The drawing under review shows one solid part. Ordinate dimensions are in mm from its lowest x, y, z. A direction names the side the tool comes from. Coordinates: 2 decimals unless noted, no trailing zeros. Write each loop counter-clockwise with the first axis right and the second up, starting at its lowest first coordinate (ties: lowest second). Pieces come first, ordered by that corner, then holes.
Q1. To check wall thickness, follow probe 1 along X at (y, z) = (65, 14); probe 2 along X at (y, z) = (1.95, 8); probe 3 along Y at (x, z) = (93.5, 11). State the ranges of each line that lie inside material, in increasing order.
Q2. Machinability: for the marked faces 1 and 2, which of the approach directions +Z, -Z, +X, -X, +Y, -Y give a long, thin tool a straight path to every point of the face, cutting with its end or side? Answer none if there is none.
Q3. Add section A-A, the plane y = 20. Give the boundary of the cut face in (x, z), plus the area to 3 significant figures.
Q4. Add section B-B, the plane x = 40.5. Give the boundary of the cut face in (y, z), plus the area to 4 significant figures.
Q5. The part is to be moulded in two halves that separate along X. For the marked faces 3, 4 and 5, say which applies: +X half, -X half, draft (parallel to the pull), parting line (faces both ways), or undercut.
Q6. Add section C-C, the plane z = 8. Give the boundary of the cut face in (x, y).
Q7. Add section D-D, the plane z = 14.25. Give the boundary of the cut face in (x, y).
Q8. Clearance check with flat-ended pins moving along their axes: pin 1 Ø2 at (x, y) = (40.5, 63) entering from -Z; pin 2 Ø10 at (x, y) = (48.5, 30.5) entering from +Z; pin 3 Ø0.9 at (x, y) = (51, 82) entering from +Z; pin 4 Ø9 at (x, z) = (103.5, 8) entering from -Y. State where each tip first meets the part, or that it passes through.
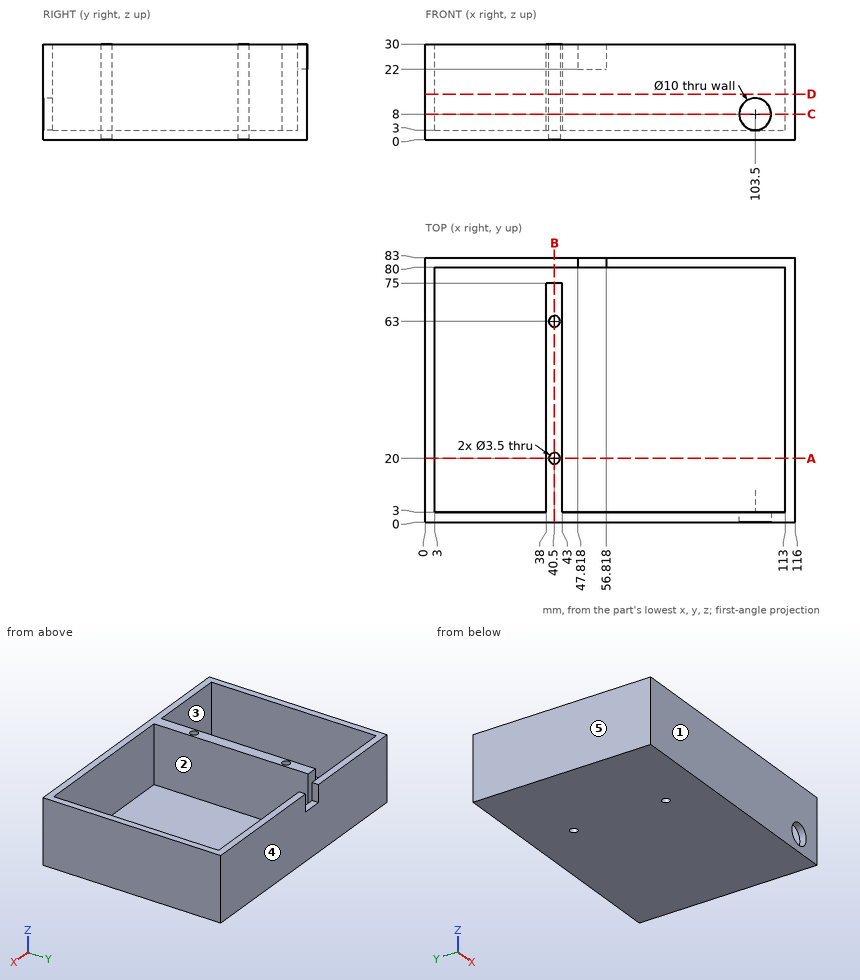
Here are the results:
1. probe 1: x = 0 to 3, 38 to 43, 113 to 116
1. probe 2: x = 0 to 98.5, 108.5 to 116
1. probe 3: y = 0 to 3, 80 to 83
2. face 1: +Z, -Z, +X, -X, -Y
2. face 2: +Z
3. outline: (0, 0) - (38.75, 0) - (38.75, 30) - (38, 30) - (38, 3) - (3, 3) - (3, 30) - (0, 30) - close; (42.25, 0) - (116, 0) - (116, 30) - (113, 30) - (113, 3) - (43, 3) - (43, 30) - (42.25, 30) - close
3. area: 540 mm2
4. outline: (0, 0) - (18.25, 0) - (18.25, 30) - (0, 30) - close; (21.75, 0) - (61.25, 0) - (61.25, 30) - (21.75, 30) - close; (64.75, 0) - (83, 0) - (83, 30) - (80, 30) - (80, 3) - (75, 3) - (75, 30) - (64.75, 30) - close
4. area: 2,145 mm2
5. face 3: undercut
5. face 4: draft
5. face 5: -X half
6. outline: (0, 0) - (98.5, 0) - (98.5, 3) - (43, 3) - (43, 75) - (38, 75) - (38, 3) - (3, 3) - (3, 80) - (113, 80) - (113, 3) - (108.5, 3) - (108.5, 0) - (116, 0) - (116, 83) - (0, 83) - close; hole circle Ø3.5 at (40.5, 20); hole circle Ø3.5 at (40.5, 63)
7. outline: (0, 0) - (116, 0) - (116, 83) - (0, 83) - close; hole (3, 3) - (38, 3) - (38, 75) - (43, 75) - (43, 3) - (113, 3) - (113, 80) - (3, 80) - close; hole circle Ø3.5 at (40.5, 20); hole circle Ø3.5 at (40.5, 63)
8. pin 1: passes through
8. pin 2: stops at z = 3
8. pin 3: stops at z = 22
8. pin 4: stops at y = 80
